Verification items for the finished model (mm, model axes). A direction names the side the tool comes from. Round coordinates to 2 decimals unless told otherwise and drop trailing zeros. Write each loop counter-clockwise with the first axis right and the second up, starting at its lowest first coordinate (ties: lowest second). Pieces come first, ordered by that corner, then holes. Notation, with made-up numbers: (-7.75, 26.25) -> (36.25, 26.25) arc R4 cw to (36.25, 31.25) -> close; hole circle Ø10 at (54.25, 74). An arc over 180 degrees is marked (long way). Use CSV: the item, a comma, the result in double quotes.
```python
from build123d import *

# Parameters (mm, degrees)
SKETCH1_W           = 50
SKETCH1_H           = 32
BOSS_EXTRUDE1_DEPTH = 47.5
SKETCH4_R           = 5
CUT_EXTRUDE1_DEPTH  = 75


with BuildPart() as part:
    # Sketch1 → Boss-Extrude1 (new, symmetric)
    with BuildSketch(Plane(origin=(0, 0, 0), x_dir=(0, 0, -1), z_dir=(1, 0, 0))):
        Rectangle(SKETCH1_W, SKETCH1_H)
    extrude(amount=BOSS_EXTRUDE1_DEPTH, both=True)

    # Sketch3 → Cut-Revolve1 (revolve, cut)
    with BuildSketch(Plane(origin=(0, 0, 0), x_dir=(0, 0, -1), z_dir=(1, 0, 0))):
        Polygon((-25, -12.35), (-11.5, -12.35), (-11.5, -7.35), (11.5, -7.35), (11.5, -12.35), (25, -12.35), (25, 16.59588936), (-25, 16.59588936), align=None)
    revolve(axis=Axis((0, 17.65, -20.249126458), (0, 0, -1)), mode=Mode.SUBTRACT)

    # Sketch4 → Cut-Extrude1 (cut)
    with BuildSketch(Plane(origin=(0, 16, 0), x_dir=(1, 0, 0), z_dir=(0, 1, 0))):
        with Locations(Location((-35, 0, 0), (0, 0, 270))):
            Circle(SKETCH4_R)
        with Locations(Location((35, 0, 0), (0, 0, 270))):
            Circle(SKETCH4_R)
    extrude(amount=-CUT_EXTRUDE1_DEPTH, mode=Mode.SUBTRACT)


solid = part.part
```
Q1. Mould release check, pull along X, two halves, no side actions. Record for faces 4 (the flat face through (0, -8, 11.5)), 5 (the flat face through (-41, 16, 0)), 6 (the flat face through (-47.5, 0, 0)): released by +X, released by -X, zero draft, split by the parting line, or undercut.
Filled in:
face 4,"undercut"
face 5,"zero draft"
face 6,"released by -X"
Q2. Access from +Z, -Z, +X, -X, +Y, -Y to the whole of each face (thin tool, end or side, straight path). Record for faces 1 (the cylindrical face through (0.637, -12.343, -18.344)), 2 (the cylindrical face through (0.637, -12.343, 18.156)), 3 (the flat face through (1, -14, 25)).
Filled in:
face 1,"-Z, +Y"
face 2,"+Z, +Y"
face 3,"+Z, +X, -X, +Y, -Y"
Q3. Go/stop test with flat-tipped pins: P1, Ø12, axis at x = -7.5, y = 7, coming from the -Z side; P2, Ø1, axis at x = 17, z = 5.5, coming from the +Y side; P3, Ø1.5, axis at x = -5.5, z = 0.5, coming from the +Y side; P4, Ø10, axis at x = -16.5, z = -1, coming from the +Y side. Record where each tip stops, or that it passes through.
Filled in:
P1,"through"
P2,"y = -0.2"
P3,"y = -6.56"
P4,"y = 4.89"
Q4. Section check A-A (y = 13.5). Record the cut outline in (x, z), plus the area to 3 significant figures.
Filled in:
outline,"(-47.5, -25) -> (-29.71, -25) -> (-29.71, -11.5) -> (-24.65, -11.5) -> (-24.65, 11.5) -> (-29.71, 11.5) -> (-29.71, 25) -> (-47.5, 25) -> close; (24.65, -11.5) -> (29.71, -11.5) -> (29.71, -25) -> (47.5, -25) -> (47.5, 25) -> (29.71, 25) -> (29.71, 11.5) -> (24.65, 11.5) -> close; hole circle Ø10 at (-35, 0); hole circle Ø10 at (35, 0)"
area,"1,850 mm²"
Q5. Section check B-B (z = 0). Record the cut outline in (x, y).
Filled in:
outline,"(-47.5, -16) -> (-40, -16) -> (-40, 16) -> (-47.5, 16) -> close; (-30, -16) -> (30, -16) -> (30, 16) -> (24.95, 16) arc R25 cw to (-24.95, 16) -> (-30, 16) -> close; (40, -16) -> (47.5, -16) -> (47.5, 16) -> (40, 16) -> close"
Q6. Section check D-D (x = 0). Record the cut outline in (y, z), plus the area to 4 significant figures.
Filled in:
outline,"(-16, -25) -> (-12.35, -25) -> (-12.35, -11.5) -> (-7.35, -11.5) -> (-7.35, 11.5) -> (-12.35, 11.5) -> (-12.35, 25) -> (-16, 25) -> close"
area,"297.5 mm²"
Q7. Material ranges on L1, parallel to X at y = 11, z = 1; L2, parallel to X at y = 7.5, z = 0; L3, parallel to Z at x = -29, y = 12, recorded low to high.
Filled in:
L1,"-47.5 to -39.9, -30.1 to -24.1, 24.1 to 30.1, 39.9 to 47.5"
L2,"-47.5 to -40, -30 to -22.85, 22.85 to 30, 40 to 47.5"
L3,"-11.5 to 11.5"
Q8. Section check C-C (x = 35). Record the cut outline in (y, z).
Filled in:
outline,"(-16, -25) -> (16, -25) -> (16, -5) -> (-16, -5) -> close; (-16, 5) -> (16, 5) -> (16, 25) -> (-16, 25) -> close"
